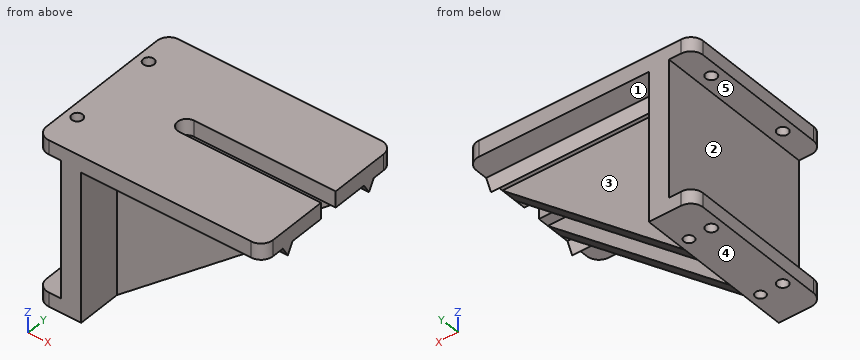
```python
from build123d import *

# Parameters (mm, degrees)
SKETCH_1_W               = 41
SKETCH_1_H               = 40
EXTRUDE_1_DEPTH          = 5
SKETCH_2_W               = 3.5
SKETCH_2_H               = 40
EXTRUDE_2_DEPTH          = 6
EXTRUDE_3_DEPTH          = 45
SKETCH_4_W               = 45
SKETCH_4_H               = 4
EXTRUDE_4_DEPTH          = 37
CUT_EXTRUDE_1_DEPTH      = 19
SKETCH_6_R               = 1.35
CUT_EXTRUDE_2_DEPTH      = 42
FILLET_1_R               = 3
FILLET_2_R               = 3
CUT_EXTRUDE_3_DEPTH      = 38
CUT_EXTRUDE_3_DEPTH_BACK = 5
SKETCH_8_R               = 1.25
CUT_EXTRUDE_4_DEPTH      = 5


with BuildPart() as part:
    # 스케치1 → 보스-돌출1 (new body)
    with BuildSketch(Plane(origin=(0, 0, 0), x_dir=(0, 0, -1), z_dir=(1, 0, 0))):
        with Locations((20.5, 20)):
            Rectangle(SKETCH_1_W, SKETCH_1_H)
    extrude(amount=EXTRUDE_1_DEPTH)

    # 스케치2 → 보스-돌출2 (add)
    with BuildSketch(Plane.ZY):
        with Locations((-1.75, 20)):
            Rectangle(SKETCH_2_W, SKETCH_2_H)
        with Locations((-39.25, 20)):
            Rectangle(SKETCH_2_W, SKETCH_2_H)
    extrude(amount=EXTRUDE_2_DEPTH)

    # 스케치3 → 보스-돌출3 (add)
    with BuildSketch(Plane(origin=(5, 0, 0), x_dir=(0, 0, -1), z_dir=(1, 0, 0))):
        Polygon((0, 40), (4, 40), (4, 34), (6.598076211, 32.5), (4, 31), (4, 14), (4, 12), (4, 9), (6.598076211, 7.5), (4, 6), (4, 0), (0, 0), align=None)
    extrude(amount=EXTRUDE_3_DEPTH)

    # 스케치4 → 보스-돌출4 (add)
    with BuildSketch(Plane(origin=(0, 0, -4), x_dir=(-1, 0, 0), z_dir=(0, 0, -1))):
        with Locations((-27.5, 27)):
            Rectangle(SKETCH_4_W, SKETCH_4_H)
        with Locations((-27.5, 13)):
            Rectangle(SKETCH_4_W, SKETCH_4_H)
    extrude(amount=EXTRUDE_4_DEPTH)

    # 스케치5 → 컷-돌출1 (cut)
    with BuildSketch(Plane(origin=(0, 29, 0), x_dir=(1, 0, 0), z_dir=(0, 1, 0))):
        Polygon((50, 4), (5, 41), (50, 41), align=None)
    extrude(amount=-CUT_EXTRUDE_1_DEPTH, mode=Mode.SUBTRACT)

    # 스케치6 → 컷-돌출2 (cut, through all)
    with BuildSketch(Plane(origin=(0, 0, -41), x_dir=(-1, 0, 0), z_dir=(0, 0, -1))):
        with Locations((3.2, 9)):
            Circle(SKETCH_6_R)
        with Locations((3.2, 31)):
            Circle(SKETCH_6_R)
    extrude(amount=-CUT_EXTRUDE_2_DEPTH, mode=Mode.SUBTRACT)

    # 필렛1
    fillet_1_edges = [part.edges().sort_by_distance(p)[0] for p in [
        (50, 0, -2),
        (50, 40, -2),
    ]]
    fillet(fillet_1_edges, radius=FILLET_1_R)

    # 필렛2
    fillet_2_edges = [part.edges().sort_by_distance(p)[0] for p in [
        (-6, 0, -1.75),
        (-6, 40, -1.75),
        (-6, 40, -39.25),
        (-6, 0, -39.25),
    ]]
    fillet(fillet_2_edges, radius=FILLET_2_R)

    # 스케치7 → 컷-돌출3 (cut, two sides)
    with BuildSketch(Plane(origin=(0, 0, -4), x_dir=(-1, 0, 0), z_dir=(0, 0, -1))) as cut_extrude_3_sk:
        with BuildLine():
            Line((-40, 22.25), (-15, 22.25))
            ThreePointArc((-15, 22.25), (-12.75, 20), (-15, 17.75))
            Line((-15, 17.75), (-40, 17.75))
            Line((-40, 17.75), (-50, 17.75))
            Line((-50, 17.75), (-50, 22.25))
            Line((-50, 22.25), (-40, 22.25))
        make_face()
    extrude(amount=CUT_EXTRUDE_3_DEPTH, mode=Mode.SUBTRACT)
    extrude(cut_extrude_3_sk.sketch, amount=-CUT_EXTRUDE_3_DEPTH_BACK, mode=Mode.SUBTRACT)

    # 스케치8 → 컷-돌출4 (cut)
    with BuildSketch(Plane(origin=(0, 0, -41), x_dir=(-1, 0, 0), z_dir=(0, 0, -1))):
        with Locations((-2.3, 31)):
            Circle(SKETCH_8_R)
        with Locations((-2.3, 9)):
            Circle(SKETCH_8_R)
    extrude(amount=-CUT_EXTRUDE_4_DEPTH, mode=Mode.SUBTRACT)


solid = part.part
```
Geometry check sheet. Reference: the model listing, model coordinates, mm. Face numbers are marked on the shaded views. A direction names the side the tool comes from. Coordinates: 2 decimals unless noted, no trailing zeros. Loops run counter-clockwise (first coordinate to the right, second up) from the corner with the lowest first, then second, coordinate; pieces in that order, holes last. Notation, with made-up numbers: (21.5, 86.25) -> (63.5, 86.25) arc R30 ccw to (63.5, 125.25) -> close; hole circle Ø8 at (62.25, 88.25). An arc over 180 degrees is marked (long way). Put each result on its own line as item: value.
1) Cross-section at D-D on y = 36. Record the boundary of the cut face in (x, z), plus the area to 3 significant figures.
Result set:
outline: (-6, -41) -> (5, -41) -> (5, -4) -> (50, -4) -> (50, 0) -> (-6, 0) -> (-6, -3.5) -> (0, -3.5) -> (0, -37.5) -> (-6, -37.5) -> close
area: 427 mm^2
2) Tool access check on the marked faces 1 and 2. Record the directions out of +Z, -Z, +X, -X, +Y, -Y that give a thin tool (end or side, any length) a straight path to the whole face; none if there is none.
Result set:
face 1: -Z, +X, +Y
face 2: -X, +Y, -Y
3) Cross-section at B-B on z = -9. Record the boundary of the cut face in (x, y).
Result set:
outline: (0, 0) -> (5, 0) -> (5, 11) -> (43.92, 11) -> (43.92, 15) -> (5, 15) -> (5, 25) -> (43.92, 25) -> (43.92, 29) -> (5, 29) -> (5, 40) -> (0, 40) -> close
4) Release check for a two-part mould opening along Z. For the marked faces 3, 4 and 5 record: released by +Z, released by -Z, zero draft, split by the parting line, or undercut.
Result set:
face 3: zero draft
face 4: released by -Z
face 5: undercut
5) Cross-section at C-C on y = 13.5. Record the boundary of the cut face in (x, z).
Result set:
outline: (-6, -41) -> (5, -41) -> (50, -4) -> (50, 0) -> (-6, 0) -> (-6, -3.5) -> (0, -3.5) -> (0, -37.5) -> (-6, -37.5) -> close
6) Thickness scan on line 1 (Y direction, x = -3.2, z = -1.75); line 2 (Y direction, x = 2.3, z = -39.05); line 3 (Y direction, x = 25, z = -3). Record the ranges inside material, lowest first.
Result set:
line 1: y = 0.01 to 7.65, 10.35 to 29.65, 32.35 to 39.99
line 2: y = 0 to 7.75, 10.25 to 29.75, 32.25 to 40
line 3: y = 0 to 17.75, 22.25 to 40
7) Cross-section at A-A on x = 2.3. Record the boundary of the cut face in (y, z), plus the area to 4 significant figures.
Result set:
outline: (0, -41) -> (7.75, -41) -> (7.75, -36) -> (10.25, -36) -> (10.25, -41) -> (29.75, -41) -> (29.75, -36) -> (32.25, -36) -> (32.25, -41) -> (40, -41) -> (40, 0) -> (0, 0) -> close
area: 1,615 mm^2
8) Gauge pin test, flat ends, axial feed: pin 1 Ø12 at (y, z) = (15, -34) entering from -X; pin 2 Ø1.2 at (x, y) = (2, 8.5) entering from -Z; pin 3 Ø5 at (x, y) = (29.5, 38) entering from -Z; pin 4 Ø5.5 at (y, z) = (3.5, -25) entering from +X. Record the tip position at first contact, or that the pin passes through.
Result set:
pin 1: stops at x = -6
pin 2: stops at z = -36
pin 3: stops at z = -4
pin 4: stops at x = 5
